The model under review builds one solid part; all positions refer to its coordinate system, in mm. A direction names the side the tool comes from. Round coordinates to 2 decimals unless told otherwise and drop trailing zeros. Loops run counter-clockwise (first coordinate to the right, second up) from the corner with the lowest first, then second, coordinate; pieces in that order, holes last. Notation, with made-up numbers: (25.25, 51) -> (31.25, 51) arc R10 ccw to (31.25, 58) -> close; hole circle Ø6 at (15, 89.5). An arc over 180 degrees is marked (long way). Write each question's results on one line, items separated by ' | '. Start each with the question number.
Item 1: We need section C-C (z = -66). Give the boundary of the cut face in (x, y).
Item 2: We need section D-D (y = -3). Give the boundary of the cut face in (x, z), and give its area (3 significant figures).
Item 3: For L1, parallel to Z at x = 0, y = -1; L2, parallel to Z at x = 94.5, y = -8.5; L3, parallel to X at y = 0, z = -8, list the stretches that pass through material, from the lowest coordinate up. Write a range as from..to.
Item 4: We need section A-A (y = 10). Give the boundary of the cut face in (x, z).
Item 5: We need section B-B (x = 0). Give the boundary of the cut face in (y, z), and give its area (3 significant figures).
Item 6: Clearance check with flat-ended pins moving along their axes: pin 1 Ø5 at (x, y) = (83, -8) entering from +Z; pin 2 Ø2 at (x, y) = (77, -1) entering from +Z; pin 3 Ø15.5 at (x, z) = (97.99, -70) entering from +Y; pin 4 Ø11 at (x, z) = (97.99, -30) entering from +Y. State where each tip first meets the part, or that it passes through.
Item 7: Mouldability with a two-part tool opening along Z and no side actions: class faces 4 (the cylindrical face through (20.16, -0.08, -19.7)), 5 (the flat face through (57.263, -0.084, 1.571)), 6 (the cylindrical face through (100.8, 0.2, -75.3)), 7 (the flat face through (11, -20.002, -11)) as pulls with the +Z half, pulls with the -Z half, needs draft (parallel to the pull), parting line crosses it, or undercut.
Item 8: Tool access review of faces 1 (the flat face through (100, -13.005, -24)), 2 (the flat face through (92, 13.005, -73)), 3 (the flat face through (100, 13.005, -24)): name each direction out of +Z, -Z, +X, -X, +Y, -Y from which nothing blocks a thin tool from reaching the whole face with its end or side.
from build123d import *

# Parameters (mm, degrees)
F1_DEPTH = 5.9944
F0_R     = 13.0048
F2_DEPTH = 20.0025
F0_R_2   = 5.9944
F3_DEPTH = 13.0048


with BuildPart() as f1:
    # F0 (on Front) → F1 (new body, symmetric)
    with BuildSketch(Plane.XZ):
        with BuildLine():
            ThreePointArc((10.294693, 22.788908), (21.008894, 13.562501), (25.0063, 0))
            ThreePointArc((25.0063, 0), (21.784516, -12.278025), (12.949346, -21.392276))
            ThreePointArc((12.949346, -21.392276), (20.268898, -19.711211), (27.152389, -22.714435))
            Line((27.152389, -22.714435), (89.990008, -78.945829))
            ThreePointArc((89.990008, -78.945829), (93.09495, -59.045979), (109.9947, -70.0024))
            Line((109.9947, -70.0024), (109.9947, -29.9974))
            ThreePointArc((109.9947, -29.9974), (87.910211, -36.506574), (102.934025, -19.060113))
            Line((102.934025, -19.060113), (10.294693, 22.788908))
        make_face()
    extrude(amount=F1_DEPTH, both=True)

    # F0 (on Front) → F2 (join, symmetric)
    with BuildSketch(Plane.XZ):
        with BuildLine():
            ThreePointArc((12.949346, -21.392276), (21.784516, -12.278025), (25.0063, 0))
            ThreePointArc((25.0063, 0), (21.008894, 13.562501), (10.294693, 22.788908))
            ThreePointArc((10.294693, 22.788908), (-24.961282, -1.499814), (12.949346, -21.392276))
        make_face()
        Circle(F0_R, mode=Mode.SUBTRACT)
    extrude(amount=F2_DEPTH, both=True)

    # F0 (on Front) → F3 (join, symmetric)
    with BuildSketch(Plane.XZ):
        with BuildLine():
            ThreePointArc((109.9947, -29.9974), (108.076189, -23.488226), (102.934025, -19.060113))
            ThreePointArc((102.934025, -19.060113), (87.910211, -36.506574), (109.9947, -29.9974))
        make_face()
        with Locations((97.9932, -29.9974)):
            Circle(F0_R_2, mode=Mode.SUBTRACT)
        with BuildLine():
            ThreePointArc((109.9947, -70.0024), (93.09495, -59.045979), (89.990008, -78.945829))
            ThreePointArc((89.990008, -78.945829), (102.89145, -80.958821), (109.9947, -70.0024))
        make_face()
        with Locations((97.9932, -70.0024)):
            Circle(F0_R_2, mode=Mode.SUBTRACT)
    extrude(amount=F3_DEPTH, both=True)


solid = f1.part
Here are the results:
1) outline: (75.52, -5.99) -> (86.68, -5.99) -> (86.68, -13) -> (93.53, -13) -> (93.53, 13) -> (86.68, 13) -> (86.68, 5.99) -> (75.52, 5.99) -> close; (102.46, -13) -> (109.31, -13) -> (109.31, -5.99) -> (109.99, -5.99) -> (109.99, 5.99) -> (109.31, 5.99) -> (109.31, 13) -> (102.46, 13) -> close
2) outline: (10.29, 22.79) arc R25.01 ccw (long way) to (12.95, -21.39) arc R11.99 cw to (27.15, -22.71) -> (89.99, -78.95) arc R12 ccw to (109.99, -70) -> (109.99, -30) arc R12 ccw to (102.93, -19.06) -> close; hole circle Ø26.01 at (0, 0); hole circle Ø11.99 at (97.99, -70); hole circle Ø11.99 at (97.99, -30) | area: 5,890 mm2
3) L1: z = -25.01..-13, 13..25.01 | L2: z = -81.48..-74.87, -65.13..-58.52, -41.48..-34.87, -25.13..-18.52 | L3: x = -23.69..-10.25, 10.25..78.45
4) outline: (10.29, 22.79) arc R25.01 ccw (long way) to (25.01, 0) arc R25.01 ccw to start; circle Ø24 at (97.99, -70); (102.93, -19.06) arc R12 ccw (long way) to (109.99, -30) arc R12 ccw to start; hole circle Ø26.01 at (0, 0); hole circle Ø11.99 at (97.99, -70); hole circle Ø11.99 at (97.99, -30)
5) outline: (-20, -25.01) -> (20, -25.01) -> (20, -13) -> (-20, -13) -> close; (-20, 13) -> (20, 13) -> (20, 25.01) -> (-20, 25.01) -> close | area: 960 mm2
6) pin 1: stops at z = -9.38 | pin 2: stops at z = -6.89 | pin 3: stops at y = 13 | pin 4: passes through
7) face 4: pulls with the -Z half | face 5: pulls with the +Z half | face 6: undercut | face 7: needs draft
8) face 1: +Z, -Z, +X, -Y | face 2: +Z, -Z, +X, -X, +Y | face 3: +Z, -Z, +X, +Y
